Geometry: final body of the model. Coordinates: model frame, mm. A direction names the side the tool comes from. Give positions to 0.01 mm unless a question says otherwise; leave off trailing zeros. Write each loop counter-clockwise with the first axis right and the second up, starting at its lowest first coordinate (ties: lowest second). Pieces come first, ordered by that corner, then holes.
Q1. Reachability of faces 4 (the face through (5, 15, -7)), 5 (the face through (21, 33, -43)), 6 (the face through (5, 84, -16)), 7 (the face through (5, 78, -71)) from +Z, -Z, +X, -X, +Y, -Y: full face, straight path, thin tool, end or side. Return the list, or none.
Q2. Pin query (flat end, axial travel): pin 1 (5.5 mm diameter, centred on x = 3.5, y = 79, fed in from -Z); pin 2 (10 mm diameter, centred on x = 28, y = 46, fed in from +Z); pin 3 (4 mm diameter, centred on x = 2.5, z = -6.5, fed in from -Y); pin 4 (10 mm diameter, centred on x = 29, z = -17, fed in from +Y). Return the tip coordinate at first contact, or that it passes through.
Q3. Draft query along Z for faces 1 (the face through (10, 81, -78)), 2 (the face through (21, 74.5, -43.3)), 3 (the face through (5, 1, -69)). Return one class per face: pulls with the +Z half, pulls with the -Z half, needs draft (parallel to the pull), parting line crosses it, or undercut.
Q4. Cut plane C-C on x = 25. Return the cut outline in (y, z).
Q5. Cut plane A-A on y = 43. Return the cut outline in (x, z).
Q6. Cut plane B-B on z = -39.5. Return the cut outline in (x, y), plus the area to 3 significant figures.
Q7. Line query: L1, parallel to Y at x = 16.5, z = -9.55; L2, parallel to Y at x = 18, z = -75.5; L3, parallel to X at y = 65.5, z = -59. Output: solid intervals per line, ascending.
```python
from build123d import *

# Parameters (mm, degrees)
BOSS_EXTRUDE1_DEPTH = 20
CUT_EXTRUDE1_DEPTH  = 10
FILLET1_R           = 5
SKETCH3_R           = 2.75
CUT_EXTRUDE2_DEPTH  = 10
SKETCH4_R           = 6
BOSS_EXTRUDE3_DEPTH = 22
SKETCH5_R           = 35
SKETCH5_R_2         = 31.5
SKETCH5_R_3         = 10
SKETCH5_R_4         = 6
BOSS_EXTRUDE4_DEPTH = 2
SKETCH6_R           = 31.5
SKETCH6_R_2         = 10
BOSS_EXTRUDE5_DEPTH = 0.1
BOSS_EXTRUDE6_DEPTH = 2


with BuildPart() as part:
    # Sketch1 → Boss-Extrude1 (new body)
    with BuildSketch(Plane(origin=(0, 0, 0), x_dir=(0, 0, -1), z_dir=(1, 0, 0))):
        with BuildLine():
            Line((8, 0), (78, 0))
            ThreePointArc((78, 0), (83.656854249, 2.343145751), (86, 8))
            Line((86, 8), (86, 78))
            ThreePointArc((86, 78), (83.656854249, 83.656854249), (78, 86))
            Line((78, 86), (8, 86))
            ThreePointArc((8, 86), (2.343145751, 83.656854249), (0, 78))
            Line((0, 78), (0, 8))
            ThreePointArc((0, 8), (2.343145751, 2.343145751), (8, 0))
        make_face()
    extrude(amount=BOSS_EXTRUDE1_DEPTH)

    # Sketch2 → Cut-Extrude1 (cut)
    with BuildSketch(Plane.ZY):
        with BuildLine():
            Line((-71, 76), (-71, 86))
            Line((-71, 86), (-78, 86))
            ThreePointArc((-78, 86), (-83.656854249, 83.656854249), (-86, 78))
            Line((-86, 78), (-86, 71))
            Line((-86, 71), (-76, 71))
            ThreePointArc((-76, 71), (-72.464466094, 72.464466094), (-71, 76))
        make_face()
        with BuildLine():
            Line((-8, 86), (-15, 86))
            Line((-15, 86), (-15, 76))
            ThreePointArc((-15, 76), (-13.535533906, 72.464466094), (-10, 71))
            Line((-10, 71), (0, 71))
            Line((0, 71), (0, 78))
            ThreePointArc((0, 78), (-2.343145751, 83.656854249), (-8, 86))
        make_face()
        with BuildLine():
            Line((0, 8), (0, 15))
            Line((0, 15), (-10, 15))
            ThreePointArc((-10, 15), (-13.535533906, 13.535533906), (-15, 10))
            Line((-15, 10), (-15, 0))
            Line((-15, 0), (-8, 0))
            ThreePointArc((-8, 0), (-2.343145751, 2.343145751), (0, 8))
        make_face()
        with BuildLine():
            Line((-76, 15), (-86, 15))
            Line((-86, 15), (-86, 8))
            ThreePointArc((-86, 8), (-83.656854249, 2.343145751), (-78, 0))
            Line((-78, 0), (-71, 0))
            Line((-71, 0), (-71, 10))
            ThreePointArc((-71, 10), (-72.464466094, 13.535533906), (-76, 15))
        make_face()
    extrude(amount=-CUT_EXTRUDE1_DEPTH, mode=Mode.SUBTRACT)

    # Fillet1
    fillet1_edges = [part.edges().sort_by_distance(p)[0] for p in [
        (5, 71, -86),
        (5, 86, -71),
        (5, 86, -15),
        (5, 71, 0),
        (5, 15, 0),
        (5, 0, -15),
        (5, 0, -71),
        (5, 15, -86),
    ]]
    fillet(fillet1_edges, radius=FILLET1_R)

    # Sketch3 → Cut-Extrude2 (cut)
    with BuildSketch(Plane(origin=(20, 0, 0), x_dir=(0, 0, -1), z_dir=(1, 0, 0))):
        with Locations((9.55, 76.45)):
            Circle(SKETCH3_R)
        with Locations((76.45, 76.45)):
            Circle(SKETCH3_R)
        with Locations((76.45, 9.55)):
            Circle(SKETCH3_R)
        with Locations((9.55, 9.55)):
            Circle(SKETCH3_R)
    extrude(amount=-CUT_EXTRUDE2_DEPTH, mode=Mode.SUBTRACT)

    # Sketch4 → Boss-Extrude3 (add)
    with BuildSketch(Plane(origin=(20, 0, 0), x_dir=(0, 0, -1), z_dir=(1, 0, 0))):
        with Locations((43, 43)):
            Circle(SKETCH4_R)
    extrude(amount=BOSS_EXTRUDE3_DEPTH)

    # Sketch5 → Boss-Extrude4 (add)
    with BuildSketch(Plane(origin=(20, 0, 0), x_dir=(0, 0, -1), z_dir=(1, 0, 0))):
        with Locations((43, 43)):
            Circle(SKETCH5_R)
        with Locations((43, 43)):
            Circle(SKETCH5_R_2, mode=Mode.SUBTRACT)
        with Locations((43, 43)):
            Circle(SKETCH5_R_3)
        with Locations((43, 43)):
            Circle(SKETCH5_R_4, mode=Mode.SUBTRACT)
    extrude(amount=BOSS_EXTRUDE4_DEPTH)

    # Sketch6 → Boss-Extrude5 (add)
    with BuildSketch(Plane(origin=(20, 0, 0), x_dir=(0, 0, -1), z_dir=(1, 0, 0))):
        with Locations((43, 43)):
            Circle(SKETCH6_R)
        with Locations((43, 43)):
            Circle(SKETCH6_R_2, mode=Mode.SUBTRACT)
    extrude(amount=BOSS_EXTRUDE5_DEPTH)

    # Sketch7 → Boss-Extrude6 (add)
    with BuildSketch(Plane(origin=(20, 0, 0), x_dir=(0, 0, -1), z_dir=(1, 0, 0))):
        Polygon((37.343145751, 50.071067812), (35.928932188, 48.656854249), (19.665476221, 64.920310217), (21.079689783, 66.334523779), align=None)
        Polygon((21.079689783, 19.665476221), (37.343145751, 35.928932188), (35.928932188, 37.343145751), (19.665476221, 21.079689783), align=None)
        Polygon((66.334523779, 21.079689783), (50.071067812, 37.343145751), (48.656854249, 35.928932188), (64.920310217, 19.665476221), align=None)
        Polygon((64.920310217, 66.334523779), (48.656854249, 50.071067812), (50.071067812, 48.656854249), (66.334523779, 64.920310217), align=None)
    extrude(amount=BOSS_EXTRUDE6_DEPTH)


solid = part.part
```
Data:
1. face 4: +Z, -X, -Y
1. face 5: +X
1. face 6: +Z, -X, +Y
1. face 7: -Z, -X, +Y
2. pin 1: stops at z = -71
2. pin 2: stops at z = -37
2. pin 3: stops at y = 15
2. pin 4: passes through
3. face 1: needs draft
3. face 2: undercut
3. face 3: pulls with the -Z half
4. outline: circle Ø12 at (43, -43)
5. outline: (0, -86) - (20, -86) - (20, -78) - (22, -78) - (22, -74.5) - (20.1, -74.5) - (20.1, -53) - (22, -53) - (22, -49) - (42, -49) - (42, -37) - (22, -37) - (22, -33) - (20.1, -33) - (20.1, -11.5) - (22, -11.5) - (22, -8) - (20, -8) - (20, 0) - (0, 0) - close
6. outline: (0, 0) - (20, 0) - (20, 8.18) - (22, 8.18) - (22, 11.7) - (20.1, 11.7) - (20.1, 33.63) - (22, 33.63) - (22, 38.13) - (42, 38.13) - (42, 47.87) - (22, 47.87) - (22, 52.37) - (20.1, 52.37) - (20.1, 74.3) - (22, 74.3) - (22, 77.82) - (20, 77.82) - (20, 86) - (0, 86) - close
6. area: 1,970 mm2
7. L1: y = 0 to 6.8, 12.3 to 73.7, 79.2 to 86
7. L2: y = 0 to 6.97, 12.13 to 73.87, 79.03 to 86
7. L3: x = 0 to 20.1
